from build123d import *

# Parameters (mm, degrees)
F0_W     = 32.5
F0_H     = 200
F2_W     = 85
F2_H     = 85
F3_DEPTH = 10
F5_W     = 85
F5_H     = 85
F6_DEPTH = 10


with BuildPart() as f1:
    # F0 (on Front) → F1 (revolve)
    with BuildSketch(Plane.XZ):
        with Locations((-16.25, 90)):
            Rectangle(F0_W, F0_H)
    revolve(axis=Axis((0, 0, 90), (0, 0, -1)))

    # F2 (on Top) → F3 (join)
    with BuildSketch(Plane.XY):
        Rectangle(F2_W, F2_H)
    extrude(amount=F3_DEPTH)

    # F5 (on offset) → F6 (join)
    with BuildSketch(Plane.XY.offset(65)):
        Rectangle(F5_W, F5_H)
    extrude(amount=-F6_DEPTH)


solid = f1.part
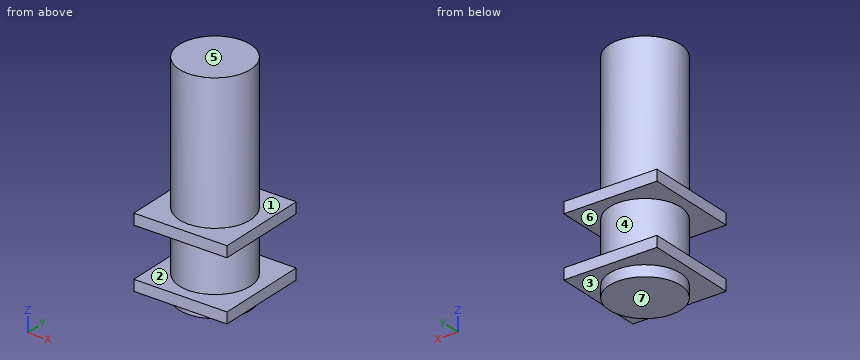
Geometry: final body of the model. Coordinates: model frame, mm. Face numbers are marked on the shaded views. A direction names the side the tool comes from. Round coordinates to 2 decimals unless told otherwise and drop trailing zeros. Order: outer loops, then holes, each group sorted by start corner. A loop starts at its lowest first (then second) coordinate and runs counter-clockwise, first axis right, second up. Notation, with made-up numbers: (87, -38.5) -> (129, -38.5) arc R24 ccw to (129, -24.5) -> close; hole circle Ø4 at (73.5, 2). An arc over 180 degrees is marked (long way). Put each result on its own line as item: value. Start each with the question number.
Q1. First-contact query: pin 1 (10 mm diameter, centred on x = 10.5, z = 135, fed in from +Y); pin 2 (2 mm diameter, centred on x = -21, z = 18.5, fed in from +Y); pin 3 (10 mm diameter, centred on y = -15.5, z = 86.5, fed in from -X). Flat tips, straight axial feed; report the tip coordinate or a pass-through.
Q2. Section D-D on z = 125.5. Return the cut outline in (x, y), and give its area (3 significant figures).
Q3. Section B-B on x = 0. Return the cut outline in (y, z).
Q4. Line query: probe 1 along Z at (x, y) = (-37, 36.5); probe 2 along Y at (x, z) = (0.5, 97); probe 3 along X at (y, z) = (28, 72). Output: solid intervals per line, ascending.
Q5. Reachability of the marked faces 1, 2 and 3 from +Z, -Z, +X, -X, +Y, -Y: full face, straight path, thin tool, end or side. Return the list, or none.
Q6. Pull-direction query (Z, two-part tool) for the marked faces 4, 5, 6 and 7; classes: +Z half, -Z half, draft (parallel to the pull), parting line (faces both ways), or undercut.
Q7. Section A-A on y = 35. Return the cut outline in (x, z).
Ans:
1. pin 1: stops at y = 32.03
1. pin 2: stops at y = 25.62
1. pin 3: stops at x = -30.76
2. outline: circle Ø65 at (0, 0)
2. area: 3,320 mm2
3. outline: (-42.5, 0) -> (-32.5, 0) -> (-32.5, -10) -> (32.5, -10) -> (32.5, 0) -> (42.5, 0) -> (42.5, 10) -> (32.5, 10) -> (32.5, 55) -> (42.5, 55) -> (42.5, 65) -> (32.5, 65) -> (32.5, 190) -> (-32.5, 190) -> (-32.5, 65) -> (-42.5, 65) -> (-42.5, 55) -> (-32.5, 55) -> (-32.5, 10) -> (-42.5, 10) -> close
4. probe 1: z = 0 to 10, 55 to 65
4. probe 2: y = -32.5 to 32.5
4. probe 3: x = -16.5 to 16.5
5. face 1: +Z
5. face 2: none
5. face 3: -Z
6. face 4: undercut
6. face 5: +Z half
6. face 6: undercut
6. face 7: -Z half
7. outline: (-42.5, 0) -> (42.5, 0) -> (42.5, 10) -> (-42.5, 10) -> close; (-42.5, 55) -> (42.5, 55) -> (42.5, 65) -> (-42.5, 65) -> close
